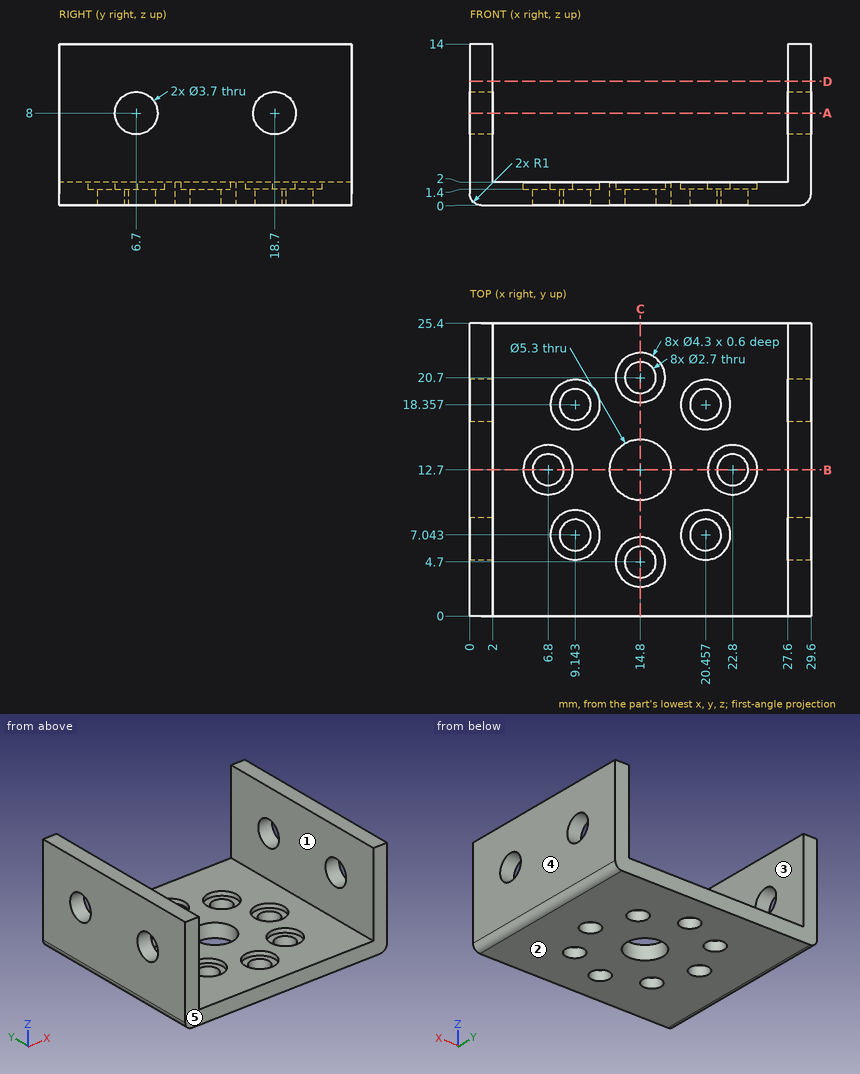
Job drawing, mm, ordinate dimensions from the low corner. One solid piece. A direction names the side the tool comes from. Round coordinates to 2 decimals unless told otherwise and drop trailing zeros. Loops run counter-clockwise (first coordinate to the right, second up) from the corner with the lowest first, then second, coordinate; pieces in that order, holes last. Notation, with made-up numbers: M 47,38 L 61,38 A18 cw 61,49 Z; hole C 73.25,36.25 d10. An arc over 180 degrees is marked long. Answer as CSV lines item,"result".
1. Flat gauge pins, fed straight in: P1, Ø4.5, axis at x = 9.5, y = 19, coming from the +Z side; P2, Ø3.5, axis at x = 20.5, y = 7, coming from the +Z side. Where does each tip first touch, or does it go through?
Resolved:
P1,"stops at z = 2"
P2,"stops at z = 1.4"
2. 3-axis set-ups, long thin cutter, end or side, ignore diameter. For the marked faces 1 and 2: which of +Z, -Z, +X, -X, +Y, -Y reach the whole face in a straight line?
Resolved:
face 1,"+Z, +Y, -Y"
face 2,"-Z, +X, -X, +Y, -Y"
3. Cut at B-B on y = 12.7. Count the separate pieces of the cut face and the enclosed holes in it.
Resolved:
separate pieces,"4"
enclosed holes,"0"
4. Wall check: probe 1 along Y at (x, z) = (14.8, 0.6); probe 2 along Y at (x, z) = (1.55, 8); probe 3 along X at (y, z) = (21.25, 12.5). Give the ranges that are in metal, low to high. Write a range as [from, to].
Resolved:
probe 1,"y = [0, 3.35], [6.05, 10.05], [15.35, 19.35], [22.05, 25.4]"
probe 2,"y = [0, 4.85], [8.55, 16.85], [20.55, 25.4]"
probe 3,"x = [0, 2], [27.6, 29.6]"
5. Two-plate mould, pull along X, no slides. Class the marked faces 3, 4 and 5: released by +X, released by -X, zero draft, split by the parting line, or undercut.
Resolved:
face 3,"undercut"
face 4,"released by +X"
face 5,"zero draft"
6. Cut at C-C on x = 14.8. Write the cut outline in (y, z).
Resolved:
outline,"M 0,0 L 3.35,0 L 3.35,1.4 L 2.55,1.4 L 2.55,2 L 0,2 Z; M 6.05,0 L 10.05,0 L 10.05,2 L 6.85,2 L 6.85,1.4 L 6.05,1.4 Z; M 15.35,0 L 19.35,0 L 19.35,1.4 L 18.55,1.4 L 18.55,2 L 15.35,2 Z; M 22.05,0 L 25.4,0 L 25.4,2 L 22.85,2 L 22.85,1.4 L 22.05,1.4 Z"
7. Cut at D-D on z = 10.75. Write the cut outline in (x, y).
Resolved:
outline,"M 0,0 L 2,0 L 2,25.4 L 0,25.4 Z; M 27.6,0 L 29.6,0 L 29.6,25.4 L 27.6,25.4 Z"
8. Cut at A-A on z = 8. Write the cut outline in (x, y), then the cut area to 3 significant figures.
Resolved:
outline,"M 0,0 L 2,0 L 2,4.85 L 0,4.85 Z; M 0,8.55 L 2,8.55 L 2,16.85 L 0,16.85 Z; M 0,20.55 L 2,20.55 L 2,25.4 L 0,25.4 Z; M 27.6,0 L 29.6,0 L 29.6,4.85 L 27.6,4.85 Z; M 27.6,8.55 L 29.6,8.55 L 29.6,16.85 L 27.6,16.85 Z; M 27.6,20.55 L 29.6,20.55 L 29.6,25.4 L 27.6,25.4 Z"
area,"72.0 mm²"
